from build123d import *

# Parameters (mm, degrees)
SKETCH3_W                = 111.348371095
SKETCH3_H                = 23.1
BOSS_EXTRUDE1_DEPTH      = 5
SKETCH3_4_W              = 34.9
SKETCH3_4_H              = 23.1
BOSS_EXTRUDE2_DEPTH      = 2.5
CUT_EXTRUDE1_DEPTH       = 30.8
CUT_EXTRUDE1_DEPTH_BACK  = 67.894637304
SKETCH4_4_R              = 12.7
BOSS_EXTRUDE3_START      = -1
SKETCH4_R                = 12.7
SKETCH4_R_2              = 4
SKETCH4_R_3              = 1.6
BOSS_EXTRUDE3_DEPTH      = 2
BOSS_EXTRUDE4_DEPTH      = 2
BOSS_EXTRUDE4_DEPTH_BACK = 13
BOSS_EXTRUDE4_START      = -3
SKETCH4_3_R              = 14.8
SKETCH4_3_R_2            = 12.7
SKETCH5_R                = 4.6
SKETCH5_R_2              = 1.6
BOSS_EXTRUDE5_DEPTH      = 5
BOSS_EXTRUDE6_START      = 11.55
SKETCH6_R                = 1.7
BOSS_EXTRUDE6_DEPTH      = 2
BOSS_EXTRUDE7_START      = -11.55
BOSS_EXTRUDE7_OUTLINE_R  = 1.7
BOSS_EXTRUDE7_DEPTH      = 2
BOSS_EXTRUDE8_DEPTH      = 2
SHELL1_START             = -5
SHELL1_DEPTH             = 0.1
SHELL1_START_2           = -4.9
SHELL1_2_DEPTH           = 2.9
SHELL1_START_3           = -97.348371095
SHELL1_3_DEPTH           = 76.448371095
SHELL1_START_4           = -56.7
SHELL1_4_DEPTH           = 2
SHELL1_START_5           = -22.9
SHELL1_5_DEPTH           = 2


with BuildPart() as part:
    # Sketch3 → Boss-Extrude1 (new body)
    with BuildSketch(Plane(origin=(0, 0, 0), x_dir=(1, 0, 0), z_dir=(0, 1, 0))):
        with Locations((-43.674185548, 0)):
            Rectangle(SKETCH3_W, SKETCH3_H)
    extrude(amount=-BOSS_EXTRUDE1_DEPTH)

    # Sketch3<4> → Boss-Extrude2 (add)
    with BuildSketch(Plane(origin=(0, 0, 0), x_dir=(1, 0, 0), z_dir=(0, 1, 0))):
        with Locations((-5.45, 0)):
            Rectangle(SKETCH3_4_W, SKETCH3_4_H)
        Polygon((-20.2, 9.55), (9.3, 9.55), (10, 9.55), (10, -9.55), (9.3, -9.55), (-20.2, -9.55), (-20.9, -9.55), (-20.9, 9.55), align=None, mode=Mode.SUBTRACT)
    extrude(amount=BOSS_EXTRUDE2_DEPTH)

    # Sketch4<4> → Cut-Extrude1 (cut, two sides: drawn at the far end of the back side and taken through both)
    with BuildSketch(Plane(origin=(-53.7, 0, 0), x_dir=(0, 0, -1), z_dir=(1, 0, 0)).offset(-CUT_EXTRUDE1_DEPTH_BACK)):
        with Locations((0, 9.8)):
            Circle(SKETCH4_4_R)
    extrude(amount=CUT_EXTRUDE1_DEPTH + CUT_EXTRUDE1_DEPTH_BACK, mode=Mode.SUBTRACT)

    # Sketch4 → Boss-Extrude3 (add)
    with BuildSketch(Plane(origin=(-53.7, 0, 0), x_dir=(0, 0, -1), z_dir=(1, 0, 0)).offset(BOSS_EXTRUDE3_START)):
        with Locations((0, 9.8)):
            Circle(SKETCH4_R)
        with Locations((0, 9.8)):
            Circle(SKETCH4_R_2, mode=Mode.SUBTRACT)
        with Locations((0, 18.3)):
            Circle(SKETCH4_R_3, mode=Mode.SUBTRACT)
        with Locations((0, 1.3)):
            Circle(SKETCH4_R_3, mode=Mode.SUBTRACT)
    extrude(amount=-BOSS_EXTRUDE3_DEPTH)

    # Sketch4<3> → Boss-Extrude4 (add, two sides: drawn at the far end of the back side and taken through both)
    with BuildSketch(Plane(origin=(-53.7, 0, 0), x_dir=(0, 0, -1), z_dir=(1, 0, 0)).offset(BOSS_EXTRUDE4_START - BOSS_EXTRUDE4_DEPTH_BACK)):
        with Locations((0, 9.8)):
            Circle(SKETCH4_3_R)
        with Locations((0, 9.8)):
            Circle(SKETCH4_3_R_2, mode=Mode.SUBTRACT)
    extrude(amount=BOSS_EXTRUDE4_DEPTH + BOSS_EXTRUDE4_DEPTH_BACK)

    # Sketch5 → Boss-Extrude5 (add)
    # profile 1 of 6: a face of its own
    with BuildSketch(Plane(origin=(0, 0, 0), x_dir=(1, 0, 0), z_dir=(0, 1, 0))):
        with Locations((-47.098371095, -16.15)):
            Circle(SKETCH5_R)
        with Locations(Location((-47.098371095, -16.15, 0), (0, 0, 270))):
            Circle(SKETCH5_R_2, mode=Mode.SUBTRACT)
    # profile 2 of 6: a face of its own
    with BuildSketch(Plane(origin=(0, 0, 0), x_dir=(1, 0, 0), z_dir=(0, 1, 0))):
        with BuildLine():
            Line((-51.698371095, -11.55), (-51.698371095, -16.15))
            ThreePointArc((-51.698371095, -16.15), (-50.351062288, -12.897308807), (-47.098371095, -11.55))
            Line((-47.098371095, -11.55), (-51.698371095, -11.55))
        make_face()
    # profile 3 of 6: a face of its own
    with BuildSketch(Plane(origin=(0, 0, 0), x_dir=(1, 0, 0), z_dir=(0, 1, 0))):
        with BuildLine():
            ThreePointArc((-47.098371095, -11.55), (-43.845679901, -12.897308807), (-42.498371095, -16.15))
            Line((-42.498371095, -16.15), (-42.498371095, -11.55))
            Line((-42.498371095, -11.55), (-47.098371095, -11.55))
        make_face()
    # profile 4 of 6: a face of its own
    with BuildSketch(Plane(origin=(0, 0, 0), x_dir=(1, 0, 0), z_dir=(0, 1, 0))):
        with Locations((-71.298371095, -16.15)):
            Circle(SKETCH5_R)
        with Locations(Location((-71.298371095, -16.15, 0), (0, 0, 270))):
            Circle(SKETCH5_R_2, mode=Mode.SUBTRACT)
    # profile 5 of 6: a face of its own
    with BuildSketch(Plane(origin=(0, 0, 0), x_dir=(1, 0, 0), z_dir=(0, 1, 0))):
        with BuildLine():
            ThreePointArc((-75.898371095, -16.15), (-74.551062288, -12.897308807), (-71.298371095, -11.55))
            Line((-71.298371095, -11.55), (-75.898371095, -11.55))
            Line((-75.898371095, -11.55), (-75.898371095, -16.15))
        make_face()
    # profile 6 of 6: a face of its own
    with BuildSketch(Plane(origin=(0, 0, 0), x_dir=(1, 0, 0), z_dir=(0, 1, 0))):
        with BuildLine():
            Line((-66.698371095, -16.15), (-66.698371095, -11.55))
            Line((-66.698371095, -11.55), (-71.298371095, -11.55))
            ThreePointArc((-71.298371095, -11.55), (-68.045679901, -12.897308807), (-66.698371095, -16.15))
        make_face()
    boss_extrude5 = extrude(amount=-BOSS_EXTRUDE5_DEPTH)

    # Sketch6 → Boss-Extrude6 (add)
    with BuildSketch(Plane.XY.offset(BOSS_EXTRUDE6_START)):
        with BuildLine():
            Line((4.55162483, 8.781583733), (-22.9, 2.5))
            Line((-22.9, 2.5), (1.21821954, 2.5))
            ThreePointArc((1.21821954, 2.5), (5.6, -0.5), (9.98178046, 2.5))
            Line((9.98178046, 2.5), (12, 2.5))
            Line((12, 2.5), (9.674058028, 6.543512575))
            ThreePointArc((9.674058028, 6.543512575), (7.481735852, 8.506863149), (4.55162483, 8.781583733))
        make_face()
        with Locations(Location((5.6, 4.2, 0), (0, 0, 180))):
            Circle(SKETCH6_R, mode=Mode.SUBTRACT)
    extrude(amount=-BOSS_EXTRUDE6_DEPTH)

    # Boss-Extrude7: read off the stored shape, not the designer's step
    # Boss-Extrude7 outline → Boss-Extrude7 (add)
    with BuildSketch(Plane.XY.offset(BOSS_EXTRUDE7_START)):
        with BuildLine():
            Line((4.55162483, 8.781583733), (-22.9, 2.5))
            Line((-22.9, 2.5), (-20.9, 2.5))
            Line((-20.9, 2.5), (-20.9, 0))
            Line((-20.9, 0), (10, 0))
            Line((10, 0), (10, 2.5))
            Line((10, 2.5), (12, 2.5))
            Line((12, 2.5), (9.674058028, 6.543512575))
            ThreePointArc((9.674058028, 6.543512575), (7.481735852, 8.506863149), (4.55162483, 8.781583733))
        make_face()
        with Locations((5.6, 4.2)):
            Circle(BOSS_EXTRUDE7_OUTLINE_R, mode=Mode.SUBTRACT)
    extrude(amount=BOSS_EXTRUDE7_DEPTH)

    # Mirror1: Boss-Extrude5 across plane
    add(boss_extrude5.mirror(Plane.XY))

    # Sketch7 → Boss-Extrude8 (add)
    with BuildSketch(Plane(origin=(0, 0, -11.55), x_dir=(-1, 0, 0), z_dir=(0, 0, -1))):
        with BuildLine():
            Line((-12, 0), (-0.4, 0))
            Line((-0.4, 0), (-0.4, 7.831593371))
            Line((-0.4, 7.831593371), (-4.55162483, 8.781583733))
            ThreePointArc((-4.55162483, 8.781583733), (-7.481735852, 8.506863149), (-9.674058028, 6.543512575))
            Line((-9.674058028, 6.543512575), (-12, 2.5))
            Line((-12, 2.5), (-12, 0))
        make_face()
        Polygon((-7.2, 6.971281292), (-4, 6.971281292), (-2.4, 4.2), (-4, 1.428718708), (-7.2, 1.428718708), (-8.8, 4.2), align=None, mode=Mode.SUBTRACT)
    extrude(amount=BOSS_EXTRUDE8_DEPTH)

    # Shell1: read off the stored shape, not the designer's step
    # Shell1 outline → Shell1 (cut)
    with BuildSketch(Plane(origin=(0, 0, 0), x_dir=(1, 0, 0), z_dir=(0, 1, 0)).offset(SHELL1_START)):
        with BuildLine():
            Line((10, -9.55), (10, 9.55))
            Line((10, 9.55), (-44.498371095, 9.55))
            Line((-44.498371095, 9.55), (-44.498371095, 13.66002008))
            ThreePointArc((-44.498371095, 13.66002008), (-47.098371095, 12.55), (-49.698371095, 13.66002008))
            Line((-49.698371095, 13.66002008), (-49.698371095, 9.55))
            Line((-49.698371095, 9.55), (-68.698371095, 9.55))
            Line((-68.698371095, 9.55), (-68.698371095, 13.66002008))
            ThreePointArc((-68.698371095, 13.66002008), (-71.298371095, 12.55), (-73.898371095, 13.66002008))
            Line((-73.898371095, 13.66002008), (-73.898371095, 9.55))
            Line((-73.898371095, 9.55), (-97.348371095, 9.55))
            Line((-97.348371095, 9.55), (-97.348371095, -9.55))
            Line((-97.348371095, -9.55), (-73.898371095, -9.55))
            Line((-73.898371095, -9.55), (-73.898371095, -13.66002008))
            ThreePointArc((-73.898371095, -13.66002008), (-71.298371095, -12.55), (-68.698371095, -13.66002008))
            Line((-68.698371095, -13.66002008), (-68.698371095, -9.55))
            Line((-68.698371095, -9.55), (-49.698371095, -9.55))
            Line((-49.698371095, -9.55), (-49.698371095, -13.66002008))
            ThreePointArc((-49.698371095, -13.66002008), (-47.098371095, -12.55), (-44.498371095, -13.66002008))
            Line((-44.498371095, -13.66002008), (-44.498371095, -9.55))
            Line((-44.498371095, -9.55), (10, -9.55))
        make_face()
    extrude(amount=SHELL1_DEPTH, mode=Mode.SUBTRACT)

    # Shell1 2 outline → Shell1 2 (cut)
    with BuildSketch(Plane(origin=(0, 0, 0), x_dir=(1, 0, 0), z_dir=(0, 1, 0)).offset(SHELL1_START_2)):
        with BuildLine():
            Line((10, -9.55), (10, 9.55))
            Line((10, 9.55), (-44.498371095, 9.55))
            Line((-44.498371095, 9.55), (-44.498371095, 13.66002008))
            ThreePointArc((-44.498371095, 13.66002008), (-47.098371095, 12.55), (-49.698371095, 13.66002008))
            Line((-49.698371095, 13.66002008), (-49.698371095, 9.55))
            Line((-49.698371095, 9.55), (-68.698371095, 9.55))
            Line((-68.698371095, 9.55), (-68.698371095, 13.66002008))
            ThreePointArc((-68.698371095, 13.66002008), (-71.298371095, 12.55), (-73.898371095, 13.66002008))
            Line((-73.898371095, 13.66002008), (-73.898371095, 9.55))
            Line((-73.898371095, 9.55), (-97.348371095, 9.55))
            Line((-97.348371095, 9.55), (-97.348371095, -9.55))
            Line((-97.348371095, -9.55), (-73.898371095, -9.55))
            Line((-73.898371095, -9.55), (-73.898371095, -13.66002008))
            ThreePointArc((-73.898371095, -13.66002008), (-71.298371095, -12.55), (-68.698371095, -13.66002008))
            Line((-68.698371095, -13.66002008), (-68.698371095, -9.55))
            Line((-68.698371095, -9.55), (-49.698371095, -9.55))
            Line((-49.698371095, -9.55), (-49.698371095, -13.66002008))
            ThreePointArc((-49.698371095, -13.66002008), (-47.098371095, -12.55), (-44.498371095, -13.66002008))
            Line((-44.498371095, -13.66002008), (-44.498371095, -9.55))
            Line((-44.498371095, -9.55), (10, -9.55))
        make_face()
    extrude(amount=SHELL1_2_DEPTH, mode=Mode.SUBTRACT)

    # Shell1 3 outline → Shell1 3 (add)
    with BuildSketch(Plane.YZ.offset(SHELL1_START_3)):
        with BuildLine():
            ThreePointArc((-2, -4.695742753), (-2.9, 0), (-2, 4.695742753))
            Line((-2, 4.695742753), (-2, 8.766413178))
            ThreePointArc((-2, 8.766413178), (-4.9, 0), (-2, -8.766413178))
            Line((-2, -8.766413178), (-2, -4.695742753))
        make_face()
    extrude(amount=SHELL1_3_DEPTH)

    # Shell1 4 outline → Shell1 4 (add)
    with BuildSketch(Plane.YZ.offset(SHELL1_START_4)):
        with BuildLine():
            Line((-2, -4.695742753), (-2, 4.695742753))
            ThreePointArc((-2, 4.695742753), (-2.9, 0), (-2, -4.695742753))
        make_face()
    extrude(amount=SHELL1_4_DEPTH)

    # Shell1 5 outline → Shell1 5 (add)
    with BuildSketch(Plane.YZ.offset(SHELL1_START_5)):
        with BuildLine():
            Line((-2, -4.695742753), (-2, 4.695742753))
            ThreePointArc((-2, 4.695742753), (-2.9, 0), (-2, -4.695742753))
        make_face()
    extrude(amount=SHELL1_5_DEPTH)


solid = part.part
Read the model definition and answer for the solid it produces. Units are mm, in the model's axes. A direction names the side the tool comes from. Coordinates: 2 decimals unless noted, no trailing zeros. Loops run counter-clockwise (first coordinate to the right, second up) from the corner with the lowest first, then second, coordinate; pieces in that order, holes last.
Q1. The mould has two halves that part along Y. Classify faces 6 (the face through (-55.69, 16.74, 0.35)), 7 (the face through (-48.518, -2.465, -16.888)), 8 (the face through (7.5, 8.5, 10.6)): +Y half, -Y half, draft (parallel to the pull), parting line (faces both ways), or undercut.
Q2. Which of the six approach directions +Z, -Z, +X, -X, +Y, -Y give full straight-line access (tool end or side, diameter ignored) to faces 1 (the face through (10, 1, 0)), 2 (the face through (-66.698, -2, 14)), 3 (the face through (-20.9, -3, 0)), 4 (the face through (6, 1.429, -13)), 5 (the face through (-69.7, 22.4, 3.4))?
Q3. Consider probe 1 along X at (y, z) = (1.5, -6.5); probe 2 along X at (y, z) = (-2.9, -16.15); probe 3 along Y at (x, z) = (-55.25, 0). Determine where each line is inside the solid, lowest interval first.
Q4. The part is cut by section B-B on x = -36. Write down the section's boundary in (y, z).
Q5. The part is cut by section C-C on y = 18.3. Write down the section's boundary in (x, z).
Q6. Each of these flat-tipped pins is pushed along its axis until it touches: pin 1 Ø14 at (x, z) = (-53, 12) entering from +Y; pin 2 Ø1.5 at (x, y) = (-59, -3.5) entering from -Z; pin 3 Ø1.5 at (x, y) = (-57, 12.5) entering from +Z. Where does it stop, or does it pass through?
Q7. The part is cut by section A-A on z = 0. Give the number of separate pieces and of enclosed holes in the cut face, and give its area (3 significant figures).
Results below:
1. face 6: undercut
1. face 7: draft
1. face 8: +Y half
2. face 1: +Y
2. face 2: +Z, -Y
2. face 3: -Y
2. face 4: -Z
2. face 5: +Z, -Z, -X, +Y
3. probe 1: x = -56.7 to -54.7, -22.9 to -20.9, 10 to 12
3. probe 2: x = -75.9 to -72.9, -69.7 to -66.7, -51.7 to -48.7, -45.5 to -42.5
3. probe 3: y = -4.9 to -0.3, 2.9 to 5.8, 13.8 to 16.7, 19.9 to 24.6
4. outline: (-5, -11.55) - (0, -11.55) - (0, -8.08) arc R12.7 cw to (0, 8.08) - (0, 11.55) - (-5, 11.55) - (-5, 9.55) - (-2, 9.55) - (-2, 8.77) arc R14.7 ccw to (-2, -8.77) - (-2, -9.55) - (-5, -9.55) - close
5. outline: (-69.7, -12.12) - (-54.7, -12.12) - (-54.7, -1.6) - (-56.7, -1.6) - (-56.7, -9.44) - (-69.7, -9.44) - close; (-69.7, 9.44) - (-56.7, 9.44) - (-56.7, 1.6) - (-54.7, 1.6) - (-54.7, 12.12) - (-69.7, 12.12) - close
6. pin 1: stops at y = 23.65
6. pin 2: stops at z = -11.55
6. pin 3: stops at z = 14.67
7. separate pieces: 4
7. enclosed holes: 0
7. area: 298 mm2
